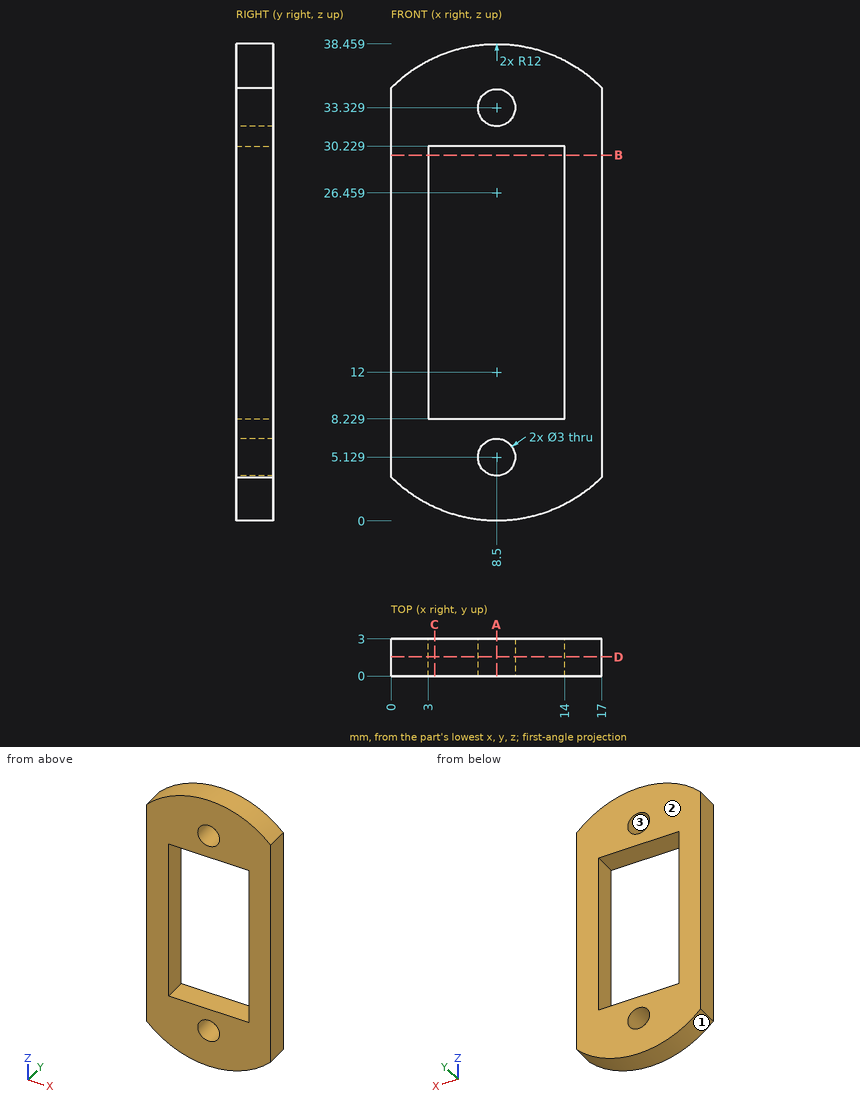
Can you work these out from the drawing? Everything is in mm from the part's minimum corner. Round coordinates to 2 decimals unless told otherwise and drop trailing zeros. Write each loop counter-clockwise with the first axis right and the second up, starting at its lowest first coordinate (ties: lowest second). Pieces come first, ordered by that corner, then holes.
1. Suppose I cut it at C-C (x = 3.5). List the corners of the cut face in (y, z) for me.
2. Suppose I cut it at D-D (y = 1.55). List the corners of the cut face in (x, z) for me.
3. Suppose I cut it at B-B (z = 29.5). List the corners of the cut face in (x, y) for me, and give its area (3 significant figures).
4. If we mould it in two halves opening along X, with no side actions, what happens to the marked faces 1, 2 and 3? For each: released by +X, released by -X, zero draft, split by the parting line, or undercut.
5. Suppose I cut it at A-A (x = 8.5). List the corners of the cut face in (y, z) for me.
6. I need wall thicknesses on L1, parallel to Z at x = 8.5, y = 0.65; L2, parallel to X at y = 0.7, z = 15.5; L3, parallel to Z at x = 8.25, y = 2.35. Which ranges of each line are inside material? Lowest first, please.
7. Will these pins go through, and if not, where does the flat tip stop? pin 1 Ø5 at (x, z) = (10, 11) entering from +Y; pin 2 Ø1.5 at (x, y) = (3.5, 2) entering from -Z; pin 3 Ø1.5 at (x, y) = (7.5, 1.5) entering from +Z.
Answer sheet:
1. outline: (0, 1.09) - (3, 1.09) - (3, 8.23) - (0, 8.23) - close; (0, 30.23) - (3, 30.23) - (3, 37.37) - (0, 37.37) - close
2. outline: (0, 3.53) arc R12 ccw to (17, 3.53) - (17, 34.93) arc R12 ccw to (0, 34.93) - close; hole (3, 8.23) - (14, 8.23) - (14, 30.23) - (3, 30.23) - close; hole circle Ø3 at (8.5, 5.13); hole circle Ø3 at (8.5, 33.33)
3. outline: (0, 0) - (3, 0) - (3, 3) - (0, 3) - close; (14, 0) - (17, 0) - (17, 3) - (14, 3) - close
3. area: 18.0 mm2
4. face 1: split by the parting line
4. face 2: zero draft
4. face 3: undercut
5. outline: (0, 0) - (3, 0) - (3, 3.63) - (0, 3.63) - close; (0, 6.63) - (3, 6.63) - (3, 8.23) - (0, 8.23) - close; (0, 30.23) - (3, 30.23) - (3, 31.83) - (0, 31.83) - close; (0, 34.83) - (3, 34.83) - (3, 38.46) - (0, 38.46) - close
6. L1: z = 0 to 3.63, 6.63 to 8.23, 30.23 to 31.83, 34.83 to 38.46
6. L2: x = 0 to 3, 14 to 17
6. L3: z = 0 to 3.65, 6.61 to 8.23, 30.23 to 31.85, 34.81 to 38.46
7. pin 1: passes through
7. pin 2: stops at z = 0.78
7. pin 3: stops at z = 38.46
